```python
from build123d import *

# Parameters (mm, degrees)
SKETCH1_R                = 13.75
BOSS_EXTRUDE1_DEPTH      = 9.5
SKETCH2_W                = 44.25
SKETCH2_H                = 20
BOSS_EXTRUDE2_DEPTH      = 9.5
BOSS_EXTRUDE3_REACH      = 49.301
BOSS_EXTRUDE3_END_RADIUS = 16.25
SKETCH3_R                = 2
SKETCH4_W                = 25
SKETCH4_H                = 7
CUT_EXTRUDE1_DEPTH       = 1


with BuildPart() as part:
    # Sketch1 → Boss-Extrude1 (new body)
    with BuildSketch(Plane(origin=(0, 0, 0), x_dir=(1, 0, 0), z_dir=(0, 1, 0))):
        with Locations(Location((0, 0, 0), (0, 0, 270))):
            Circle(SKETCH1_R)
    extrude(amount=BOSS_EXTRUDE1_DEPTH)

    # Sketch2 → Boss-Extrude2 (add)
    with BuildSketch(Plane(origin=(0, 0, 0), x_dir=(1, 0, 0), z_dir=(0, 1, 0))):
        with Locations((22.125, 0)):
            Rectangle(SKETCH2_W, SKETCH2_H)
    extrude(amount=BOSS_EXTRUDE2_DEPTH)

    # Boss-Extrude3: up to this cylinder (the profile starts inside it)
    boss_extrude3_end = Plane(origin=(0, 4.5, 0), z_dir=(0, -1, 0)) * Cylinder(BOSS_EXTRUDE3_END_RADIUS, 132.102, mode=Mode.PRIVATE)
    # Sketch3 → Boss-Extrude3 (add, up to the surface)
    with BuildSketch(Plane(origin=(0, 0, 0), x_dir=(0, 0, -1), z_dir=(1, 0, 0)), mode=Mode.PRIVATE) as boss_extrude3_sk1:
        with Locations((0, 4.5)):
            Circle(SKETCH3_R)
    boss_extrude3_tool1 = extrude(boss_extrude3_sk1.sketch, amount=-BOSS_EXTRUDE3_REACH, mode=Mode.PRIVATE) & boss_extrude3_end
    add(boss_extrude3_tool1.solids().sort_by_distance((0, 4.5, 0))[0])

    # Sketch4 → Cut-Extrude1 (cut)
    with BuildSketch(Plane(origin=(0, 9.5, 0), x_dir=(1, 0, 0), z_dir=(0, 1, 0))):
        with Locations((26.75, 0)):
            Rectangle(SKETCH4_W, SKETCH4_H)
    extrude(amount=-CUT_EXTRUDE1_DEPTH, mode=Mode.SUBTRACT)


solid = part.part
```
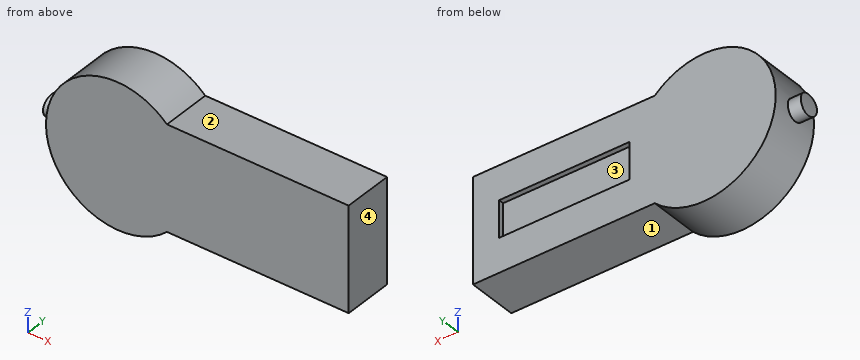
Design review of the part built by this model. Coordinates are the model's own, in mm. Face numbers are marked on the shaded views. A direction names the side the tool comes from. Coordinates: 2 decimals unless noted, no trailing zeros. Order: outer loops, then holes, each group sorted by start corner. A loop starts at its lowest first (then second) coordinate and runs counter-clockwise, first axis right, second up. Notation, with made-up numbers: (45.5, -36.5) -> (79.5, -36.5) arc R26 ccw to (79.5, 2.5) -> close; hole circle Ø6 at (31.5, 64.5). An arc over 180 degrees is marked (long way). One line per item, written item: value. Start each with the question number.
Q1. Take a section at D-D, the plane y = 1.25. State the section outline as (x, z) points.
Q2. Take a section at C-C, the plane x = 37.5. State the section outline as (y, z) points.
Q3. Insertion check: pin 1 Ø0.8 at (x, y) = (23, 9) entering from -Z; pin 2 Ø1 at (x, y) = (28.5, 6.5) entering from +Z; pin 3 Ø3.5 at (x, z) = (22.5, 1) entering from +Y. Each pin has a flat end and moves straight along its axis. Give the tip position at first contact, or say it passes through.
Q4. Take a section at A-A, the plane z = 0. State the section outline as (x, y) points.
Q5. For probe 1 along Z at (x, y) = (32, 8.75); probe 2 along Z at (x, y) = (40, 5); probe 3 along Y at (x, z) = (22.5, -2), list the stretches that pass through material, from the lowest coordinate up.
Q6. Tool access review of the marked faces 1, 2, 3 and 4: name each direction out of +Z, -Z, +X, -X, +Y, -Y from which nothing blocks a thin tool from reaching the whole face with its end or side.
Q7. Take a section at B-B, the plane y = 4.5. State the section outline as (x, z) points, then the cut area to 3 significant figures.
Values follow:
1. outline: (9.44, -10) -> (44.25, -10) -> (44.25, 10) -> (9.44, 10) arc R13.75 ccw (long way) to start
2. outline: (0, -10) -> (9.5, -10) -> (9.5, -3.5) -> (8.5, -3.5) -> (8.5, 3.5) -> (9.5, 3.5) -> (9.5, 10) -> (0, 10) -> close
3. pin 1: stops at z = -10
3. pin 2: stops at z = 10
3. pin 3: stops at y = 8.5
4. outline: (-16.25, 2.5) -> (-13.75, 2.5) -> (-13.75, 0) -> (44.25, 0) -> (44.25, 9.5) -> (39.25, 9.5) -> (39.25, 8.5) -> (14.25, 8.5) -> (14.25, 9.5) -> (-13.75, 9.5) -> (-13.75, 6.5) -> (-16.25, 6.5) -> close
5. probe 1: z = -10 to -3.5, 3.5 to 10
5. probe 2: z = -10 to 10
5. probe 3: y = 0 to 8.5
6. face 1: -Z, +X, +Y, -Y
6. face 2: +Z, +X, +Y, -Y
6. face 3: +Y
6. face 4: +Z, -Z, +X, +Y, -Y
7. outline: (-16.13, -2) -> (-13.6, -2) arc R13.75 ccw to (9.44, -10) -> (44.25, -10) -> (44.25, 10) -> (9.44, 10) arc R13.75 ccw to (-13.6, 2) -> (-16.13, 2) arc R16.25 ccw to start
7. area: 1,240 mm2
